from build123d import *

# Parameters (mm, degrees)
EXTRUDE_1_DEPTH     = 4
CUT_EXTRUDE_1_DEPTH = 10
SKETCH_3_R          = 2.25
CUT_EXTRUDE_2_DEPTH = 10
SKETCH_4_R          = 1.65
CUT_EXTRUDE_3_DEPTH = 10
SKETCH_5_R          = 2.25
SKETCH_5_W          = 40
SKETCH_5_H          = 20
CUT_EXTRUDE_4_DEPTH = 10
CUT_EXTRUDE_6_DEPTH = 10
CUT_EXTRUDE_START   = -10
CUT_EXTRUDE_7_DEPTH = 10


with BuildPart() as part:
    # 草图1 → 凸台-拉伸1 (new body)
    with BuildSketch(Plane(origin=(0, 0, 0), x_dir=(1, 0, 0), z_dir=(0, 1, 0))):
        with BuildLine():
            Line((-50, 0), (50, 0))
            ThreePointArc((50, 0), (0, -50), (-50, 0))
        make_face()
    extrude(amount=EXTRUDE_1_DEPTH)

    # 草图2 → 切除-拉伸1 (cut)
    with BuildSketch(Plane(origin=(0, 4, 0), x_dir=(1, 0, 0), z_dir=(0, 1, 0))):
        Polygon((0, -10.623043888), (10, -10.623043888), (10, -30.623043888), (-30, -30.623043888), (-30, -10.623043888), align=None)
    extrude(amount=-CUT_EXTRUDE_1_DEPTH, mode=Mode.SUBTRACT)

    # 草图3 → 切除-拉伸2 (cut)
    with BuildSketch(Plane(origin=(0, 4, 0), x_dir=(1, 0, 0), z_dir=(0, 1, 0))):
        with Locations(Location((-34.75, -15.623043888, 0), (0, 0, 270))):
            Circle(SKETCH_3_R)
        with Locations(Location((-34.75, -25.623043888, 0), (0, 0, 270))):
            Circle(SKETCH_3_R)
        with Locations(Location((14.75, -25.623043888, 0), (0, 0, 90))):
            Circle(SKETCH_3_R)
        with Locations(Location((14.75, -15.623043888, 0), (0, 0, 90))):
            Circle(SKETCH_3_R)
    extrude(amount=-CUT_EXTRUDE_2_DEPTH, mode=Mode.SUBTRACT)

    # 草图4 → 切除-拉伸3 (cut)
    with BuildSketch(Plane(origin=(0, 4, 0), x_dir=(1, 0, 0), z_dir=(0, 1, 0))):
        with Locations(Location((0, -3, 0), (0, 0, 270))):
            Circle(SKETCH_4_R)
        with Locations(Location((8, -3, 0), (0, 0, 270))):
            Circle(SKETCH_4_R)
        with Locations(Location((16, -3, 0), (0, 0, 270))):
            Circle(SKETCH_4_R)
        with Locations(Location((24, -3, 0), (0, 0, 270))):
            Circle(SKETCH_4_R)
        with Locations(Location((32, -3, 0), (0, 0, 270))):
            Circle(SKETCH_4_R)
        with Locations(Location((40, -3, 0), (0, 0, 270))):
            Circle(SKETCH_4_R)
        with Locations(Location((-40, -3, 0), (0, 0, 90))):
            Circle(SKETCH_4_R)
        with Locations(Location((-32, -3, 0), (0, 0, 90))):
            Circle(SKETCH_4_R)
        with Locations(Location((-24, -3, 0), (0, 0, 90))):
            Circle(SKETCH_4_R)
        with Locations(Location((-16, -3, 0), (0, 0, 90))):
            Circle(SKETCH_4_R)
        with Locations(Location((-8, -3, 0), (0, 0, 90))):
            Circle(SKETCH_4_R)
    extrude(amount=-CUT_EXTRUDE_3_DEPTH, mode=Mode.SUBTRACT)

    # 草图5 → 切除-拉伸4 (cut)
    with BuildSketch(Plane(origin=(0, 4, 0), x_dir=(1, 0, 0), z_dir=(0, 1, 0))):
        with BuildLine():
            Line((49.355850717, -8), (0, -8))
            Line((0, -8), (-49.355850717, -8))
            ThreePointArc((-49.355850717, -8), (0, -50), (49.355850717, -8))
        make_face()
        with Locations((-34.75, -25.623043888)):
            Circle(SKETCH_5_R, mode=Mode.SUBTRACT)
        with Locations((-10, -20.623043888)):
            Rectangle(SKETCH_5_W, SKETCH_5_H, mode=Mode.SUBTRACT)
        with Locations((-34.75, -15.623043888)):
            Circle(SKETCH_5_R, mode=Mode.SUBTRACT)
        with Locations((14.75, -25.623043888)):
            Circle(SKETCH_5_R, mode=Mode.SUBTRACT)
        with Locations((14.75, -15.623043888)):
            Circle(SKETCH_5_R, mode=Mode.SUBTRACT)
    extrude(amount=-CUT_EXTRUDE_4_DEPTH, mode=Mode.SUBTRACT)

    # 草图7 → 切除-拉伸6 (cut)
    with BuildSketch(Plane(origin=(0, 0, 0), x_dir=(-1, 0, 0), z_dir=(0, 0, -1))):
        Polygon((-50, 4), (-50, 3), (50, 3), (50, 4), (49.677925359, 4), align=None)
    extrude(amount=-CUT_EXTRUDE_6_DEPTH, mode=Mode.SUBTRACT)

    # 草图8 → 切除-拉伸7 (cut)
    with BuildSketch(Plane(origin=(0, 3, 0), x_dir=(1, 0, 0), z_dir=(0, 1, 0)).offset(CUT_EXTRUDE_START)):
        with BuildLine():
            Line((49.638694584, -6), (0, -6))
            Line((0, -6), (-49.638694584, -6))
            ThreePointArc((-49.638694584, -6), (-49.507373187, -7.001428437), (-49.355850717, -8))
            Line((-49.355850717, -8), (49.355850717, -8))
            ThreePointArc((49.355850717, -8), (49.507373187, -7.001428437), (49.638694584, -6))
        make_face()
    extrude(amount=CUT_EXTRUDE_7_DEPTH, mode=Mode.SUBTRACT)


solid = part.part
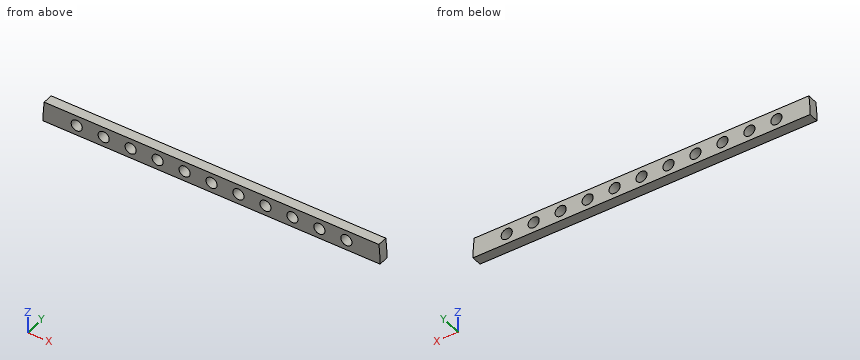
For this review, take the finished solid that the model builds, in its own axes (mm). Round coordinates to 2 decimals unless told otherwise and drop trailing zeros. Loops run counter-clockwise (first coordinate to the right, second up) from the corner with the lowest first, then second, coordinate; pieces in that order, holes last. Notation, with made-up numbers: (68, 72.25) - (110, 72.25) arc R26 ccw to (110, 89.25) - close; hole circle Ø9 at (23, 68.5). An arc over 180 degrees is marked (long way). One line per item, written item: value. Start each with the question number.
Item 1: Take a section at B-B (y = 2.55). State how many separate pieces and enclosed holes the cut face has, plus the area to 3 significant figures.
Item 2: Clearance check with a flat-ended pin moving along its axis: pin 1 Ø2.5 at (x, z) = (8, 3) entering from -Y. State where the tip first meets the part, or that it passes through.
Item 3: Take a section at A-A (x = -24). Give the boundary of the cut face in (y, z).
Item 4: For L1, parallel to Z at x = -24, y = 1.5; L2, parallel to Z at x = 23, y = 0.8; L3, parallel to X at y = 1.3, z = 0.95, list the stretches that pass through material, from the lowest coordinate up.
Answer below:
1. separate pieces: 1
1. enclosed holes: 11
1. area: 504 mm2
2. pin 1: passes through
3. outline: (0, 0) - (3, 0) - (3, 1.35) - (0, 1.35) - close; (0, 4.65) - (3, 4.65) - (3, 6) - (0, 6) - close
4. L1: z = 0 to 1.35, 4.65 to 6
4. L2: z = 0 to 1.69, 4.31 to 6
4. L3: x = -49.99 to 49.99
